Geometry: final body of the model. Coordinates: model frame, mm. A direction names the side the tool comes from. Round coordinates to 2 decimals unless told otherwise and drop trailing zeros. Loops run counter-clockwise (first coordinate to the right, second up) from the corner with the lowest first, then second, coordinate; pieces in that order, holes last. Notation, with made-up numbers: M -33.75,-20 L -2.75,-20 A5 ccw -2.75,-13 Z; hole C -7,46 d2. An arc over 180 degrees is marked long. Write each question's results on one line, items separated by ' | '.
```python
from build123d import *

# Parameters (mm, degrees)
CROQUIS1_R                        = 3.175
SALIENTE_EXTRUIR1_DEPTH           = 5
CROQUIS2_W                        = 13
CROQUIS2_H                        = 6.35
SALIENTE_EXTRUIR2_DEPTH           = 13.5
CORTAR_EXTRUIR2_REACH             = 5.175
CROQUIS5_W                        = 3.175
CROQUIS5_H                        = 2.5
CORTAR_EXTRUIR2_DIRECTION_2_REACH = 5.175
CORTAR_EXTRUIR6_REACH             = 8.35
CORTAR_EXTRUIR7_DEPTH             = 6.35
CORTAR_EXTRUIR8_DEPTH             = 13


with BuildPart() as part:
    # Croquis1 → Saliente-Extruir1 (new body)
    with BuildSketch(Plane.XY):
        Circle(CROQUIS1_R)
    extrude(amount=SALIENTE_EXTRUIR1_DEPTH)

    # Croquis2 → Saliente-Extruir2 (add)
    with BuildSketch(Plane.XY.offset(5)):
        Rectangle(CROQUIS2_W, CROQUIS2_H)
    extrude(amount=SALIENTE_EXTRUIR2_DEPTH)

    # Croquis5 → Cortar-Extruir2 (cut, up to next)
    with BuildSketch(Plane(origin=(0, 0, 0), x_dir=(1, 0, 0), z_dir=(0, 1, 0)), mode=Mode.PRIVATE) as cortar_extruir2_sk1:
        with Locations((1.5875, -1.25)):
            Rectangle(CROQUIS5_W, CROQUIS5_H)
    cortar_extruir2_tool1 = extrude(cortar_extruir2_sk1.sketch, amount=-CORTAR_EXTRUIR2_REACH, mode=Mode.PRIVATE) & part.part
    add(cortar_extruir2_tool1.solids().sort_by_distance((1.5875, 0, 1.25))[0], mode=Mode.SUBTRACT)

    # Croquis5 → Cortar-Extruir2 direction 2 (cut, up to next)
    with BuildSketch(Plane(origin=(0, 0, 0), x_dir=(1, 0, 0), z_dir=(0, 1, 0)), mode=Mode.PRIVATE) as cortar_extruir2_direction_2_sk1:
        with Locations((1.5875, -1.25)):
            Rectangle(CROQUIS5_W, CROQUIS5_H)
    cortar_extruir2_direction_2_tool1 = extrude(cortar_extruir2_direction_2_sk1.sketch, amount=CORTAR_EXTRUIR2_DIRECTION_2_REACH, mode=Mode.PRIVATE) & part.part
    add(cortar_extruir2_direction_2_tool1.solids().sort_by_distance((1.5875, 0, 1.25))[0], mode=Mode.SUBTRACT)

    # Croquis7 → Cortar-Extruir6 (cut, up to next)
    with BuildSketch(Plane(origin=(0, 3.175, 0), x_dir=(1, 0, 0), z_dir=(0, 1, 0)), mode=Mode.PRIVATE) as cortar_extruir6_sk1:
        Polygon((-3.175, -18.5), (3.175, -18.5), (3.175, -8.5), (0, -6.666912895), (-3.175, -8.5), align=None)
    cortar_extruir6_tool1 = extrude(cortar_extruir6_sk1.sketch, amount=-CORTAR_EXTRUIR6_REACH, mode=Mode.PRIVATE) & part.part
    add(cortar_extruir6_tool1.solids().sort_by_distance((0, 3.175, 13.028903))[0], mode=Mode.SUBTRACT)

    # Croquis8 → Cortar-Extruir7 (cut)
    with BuildSketch(Plane(origin=(0, 3.175, 0), x_dir=(1, 0, 0), z_dir=(0, 1, 0))):
        with BuildLine():
            Line((-6.5, -5), (-3.175, -5))
            ThreePointArc((-3.175, -5), (-5.526130047, -5.973869953), (-6.5, -8.325))
            Line((-6.5, -8.325), (-6.5, -5))
        make_face()
    cortar_extruir7 = extrude(amount=-CORTAR_EXTRUIR7_DEPTH, mode=Mode.SUBTRACT)

    # Simetría1: Cortar-Extruir7 across plane
    add(cortar_extruir7.mirror(Plane(origin=(0, 0, 0), x_dir=(0, 0, 1), z_dir=(1, 0, 0))), mode=Mode.SUBTRACT)

    # Croquis9 → Cortar-Extruir8 (cut)
    with BuildSketch(Plane(origin=(6.5, 0, 0), x_dir=(0, 0, -1), z_dir=(1, 0, 0))):
        with BuildLine():
            Line((-15.336857856, 1.19003001), (-13.785980552, 0))
            Line((-13.785980552, 0), (-15.336857856, -1.19003001))
            ThreePointArc((-15.336857856, -1.19003001), (-17.75, 0), (-15.336857856, 1.19003001))
        make_face()
    extrude(amount=-CORTAR_EXTRUIR8_DEPTH, mode=Mode.SUBTRACT)


solid = part.part
```
1. Section B-B (z = 16.25). Output: boundary loops of the cut face in (x, y) (3 decimals), then the cut area to 3 significant figures.
Answer key:
outline: M -6.5,-3.175 L -3.175,-3.175 L -3.175,-1.5 L -6.5,-1.5 Z; M -6.5,1.5 L -3.175,1.5 L -3.175,3.175 L -6.5,3.175 Z; M 3.175,-3.175 L 6.5,-3.175 L 6.5,-1.5 L 3.175,-1.5 Z; M 3.175,1.5 L 6.5,1.5 L 6.5,3.175 L 3.175,3.175 Z | area: 22.3 mm²
2. Section D-D (x = -4.25). Output: boundary loops of the cut face in (y, z) (3 decimals).
Answer key:
outline: M -3.175,5.179 L 3.175,5.179 L 3.175,18.5 L -3.175,18.5 Z; hole M -1.19,15.337 L 0,13.786 L 1.19,15.337 A1.5 ccw long Z
3. Section A-A (z = 11.5). Output: boundary loops of the cut face in (x, y) (3 decimals).
Answer key:
outline: M -6.5,-3.175 L -3.175,-3.175 L -3.175,3.175 L -6.5,3.175 Z; M 3.175,-3.175 L 6.5,-3.175 L 6.5,3.175 L 3.175,3.175 Z
4. Draft query along Z for faces 4 (the face through (-4.81, 0.6, 14.57)), 5 (the face through (-3.175, 0, 13)), 6 (the face through (2, 3, 5)), 7 (the face through (4.86, 0.6, 14.57)). Return one class per face: pulls with the +Z half, pulls with the -Z half, needs draft (parallel to the pull), parting line crosses it, or undercut.
Answer key:
face 4: undercut | face 5: needs draft | face 6: pulls with the -Z half | face 7: undercut
5. Access query for faces 1 (the face through (-3, 2, 5)), 2 (the face through (3, -3, 5)), 3 (the face through (1.61, 0.044, 7.596)). Directions: +Z, -Z, +X, -X, +Y, -Y. A direction counts if a zero-diameter tool reaches every point of the face in a straight line with its end or side. Return the directions, or none.
Answer key:
face 1: -Z, -X, +Y | face 2: -Z, +X, -Y | face 3: +Z, +Y, -Y
6. Section C-C (y = 0.75). Output: boundary loops of the cut face in (x, z) (3 decimals).
Answer key:
outline: M -6.5,8.325 A3.325 ccw -3.175,5 L -3.085,5 L -3.085,0 L 0,0 L 0,2.5 L 3.085,2.5 L 3.085,5 L 3.175,5 A3.325 ccw 6.5,8.325 L 6.5,14.763 L 3.175,14.763 L 3.175,8.5 L 0,6.667 L -3.175,8.5 L -3.175,14.763 L -6.5,14.763 Z; M -6.5,17.549 L -3.175,17.549 L -3.175,18.5 L -6.5,18.5 Z; M 3.175,17.549 L 6.5,17.549 L 6.5,18.5 L 3.175,18.5 Z
7. Pin query (flat end, axial travel): P1, Ø1.6, axis at x = 2, y = -1.5, coming from the -Z side. Return the tip coordinate at first contact, or that it passes through.
Answer key:
P1: stops at z = 2.5
8. Ray query, probe 1 along Y at (x, z) = (4.5, 16.25) (3 decimals); probe 2 along X at (y, z) = (-1.75, 15) (3 decimals); probe 3 along Z at (x, y) = (4.75, 0.5). Return the intervals inside material, ascending.
Answer key:
probe 1: y = -3.175 to -1.5, 1.5 to 3.175 | probe 2: x = -6.5 to -3.175, 3.175 to 6.5 | probe 3: z = 5.4 to 14.44, 17.66 to 18.5
